from build123d import *

# Parameters (mm, degrees)
SKETCH1_W           = 127
SKETCH1_H           = 127
BOSS_EXTRUDE1_DEPTH = 3.175
SKETCH2_R           = 11.1125
CUT_EXTRUDE1_DEPTH  = 3.175
SKETCH4_R           = 4.7625
CUT_EXTRUDE3_DEPTH  = 3.175


with BuildPart() as part:
    # Sketch1 → Boss-Extrude1 (new body)
    with BuildSketch(Plane.XY):
        Rectangle(SKETCH1_W, SKETCH1_H)
    extrude(amount=BOSS_EXTRUDE1_DEPTH)

    # Sketch2 → Cut-Extrude1 (cut)
    with BuildSketch(Plane(origin=(0, 0, 0), x_dir=(-1, 0, 0), z_dir=(0, 0, -1))):
        with Locations((0, 25.4)):
            Circle(SKETCH2_R)
        with Locations((0, -25.4)):
            Circle(SKETCH2_R)
    extrude(amount=-CUT_EXTRUDE1_DEPTH, mode=Mode.SUBTRACT)

    # Sketch4 → Cut-Extrude3 (cut)
    with BuildSketch(Plane(origin=(0, 0, 0), x_dir=(-1, 0, 0), z_dir=(0, 0, -1))):
        with Locations((52.3875, 52.3875)):
            Circle(SKETCH4_R)
        with Locations(Location((52.3875, -52.3875, 0), (0, 0, 180))):
            Circle(SKETCH4_R)
        with Locations(Location((-52.3875, 52.3875, 0), (0, 0, 180))):
            Circle(SKETCH4_R)
        with Locations((-52.3875, -52.3875)):
            Circle(SKETCH4_R)
    extrude(amount=-CUT_EXTRUDE3_DEPTH, mode=Mode.SUBTRACT)


solid = part.part
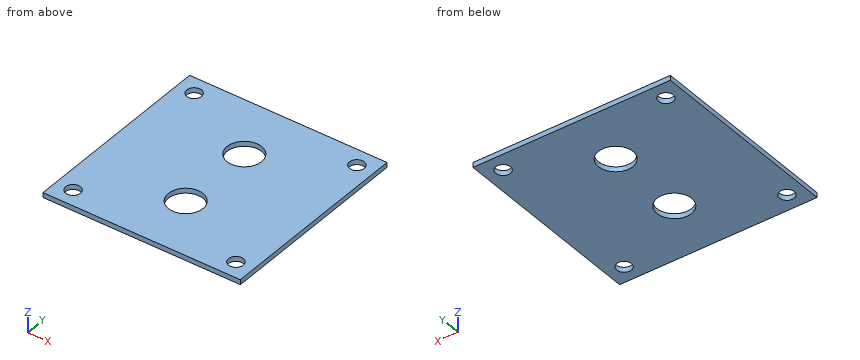
Verification items for the finished model (mm, model axes). Round coordinates to 2 decimals unless told otherwise and drop trailing zeros. Loops run counter-clockwise (first coordinate to the right, second up) from the corner with the lowest first, then second, coordinate; pieces in that order, holes last. Notation, with made-up numbers: (42, -27.5) - (65, -27.5) arc R16 cw to (65, -14.5) - close; hole circle Ø5 at (-25, 25.5). An arc over 180 degrees is marked (long way). Answer in a Markdown table with one row per item. Add a question column.
Q1. Section check B-B on x = 0. Enter the section's corners in (y, z) (1 decimal), plus the area to 3 significant figures.
Q2. Section check C-C on z = 0.55. State how many separate pieces and enclosed holes the cut face has, plus the area to 3 significant figures.
Q3. Material ranges on line 1 (Y direction, x = 0, z = 1.3); line 2 (X direction, y = 52.5, z = 1.45); line 3 (X direction, y = 49, z = 2.45), recorded low to high.
Q4. Section check A-A on y = -25.4. Enter the section's corners in (x, z) (1 decimal).
Q5. Gauge pin test, flat end, axial feed: pin 1 (5.5 mm diameter, centred on x = 52.39, y = -52.39, fed in from +Z). Record the tip position at first contact, or that the pin passes through.
Found:
| question | item | result |
|---|---|---|
| 1 | outline | (-63.5, 0) - (-36.5, 0) - (-36.5, 3.2) - (-63.5, 3.2) - close; (-14.3, 0) - (14.3, 0) - (14.3, 3.2) - (-14.3, 3.2) - close; (36.5, 0) - (63.5, 0) - (63.5, 3.2) - (36.5, 3.2) - close |
| 1 | area | 262 mm² |
| 2 | separate pieces | 1 |
| 2 | enclosed holes | 6 |
| 2 | area | 15,100 mm² |
| 3 | line 1 | y = -63.5 to -36.51, -14.29 to 14.29, 36.51 to 63.5 |
| 3 | line 2 | x = -63.5 to -57.15, -47.63 to 47.63, 57.15 to 63.5 |
| 3 | line 3 | x = -63.5 to -55.74, -49.04 to 49.04, 55.74 to 63.5 |
| 4 | outline | (-63.5, 0) - (-11.1, 0) - (-11.1, 3.2) - (-63.5, 3.2) - close; (11.1, 0) - (63.5, 0) - (63.5, 3.2) - (11.1, 3.2) - close |
| 5 | pin 1 | passes through |
